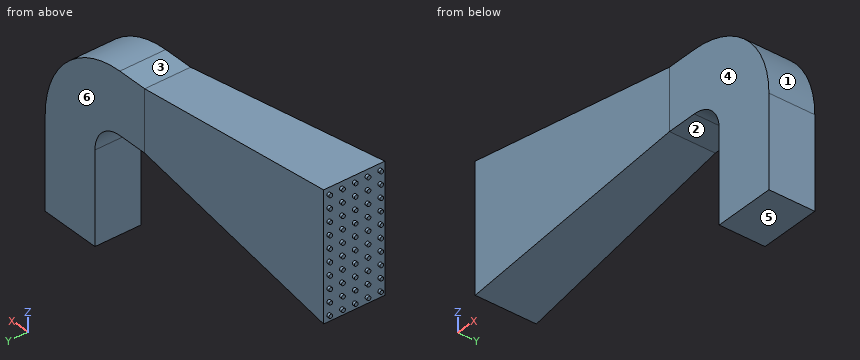
```python
from build123d import *

# Parameters (mm, degrees)
SKETCH_2_5_W    = 240
SKETCH_2_5_H    = 180
EXTRUDE_2_DEPTH = 120
SKETCH_10_W     = 240
SKETCH_10_H     = 180
REVOLVE_2_ANGLE = 90
SKETCH_11_W     = 240
SKETCH_11_H     = 180
EXTRUDE_3_DEPTH = 360
SKETCH_13_R     = 7.5
EXTRUDE_4_DEPTH = 10


with BuildPart() as part:
    # Sketch 2 → Loft 1 section 0
    with BuildSketch(Plane(origin=(900, 0, 0), x_dir=(0, 0, -1), z_dir=(1, 0, 0))):
        with BuildLine():
            Line((-120, 90), (120, 90))
            Line((120, 90), (120, -90))
            Line((120, -90), (-120, -90))
            Line((-120, -90), (-120, 90))
        make_face()
    # Sketch 1 → Loft 1 section 1
    with BuildSketch(Plane(origin=(0, 0, 0), x_dir=(0, 0, -1), z_dir=(1, 0, 0))):
        with BuildLine():
            Line((-250, 120), (250, 120))
            Line((250, 120), (250, -120))
            Line((250, -120), (-250, -120))
            Line((-250, -120), (-250, 120))
        make_face()
    loft()

    # Sketch 2_5 → Extrude 2 (add)
    with BuildSketch(Plane(origin=(900, 0, 0), x_dir=(0, 0, -1), z_dir=(1, 0, 0))):
        Rectangle(SKETCH_2_5_W, SKETCH_2_5_H)
    extrude(amount=EXTRUDE_2_DEPTH)

    # Sketch 10 → Revolve 2 (revolve)
    with BuildSketch(Plane(origin=(1020, 0, 0), x_dir=(0, 0, -1), z_dir=(1, 0, 0))):
        Rectangle(SKETCH_10_W, SKETCH_10_H)
    revolve(axis=Axis((1020, 90, -240), (0, 1, 0)), revolution_arc=REVOLVE_2_ANGLE)

    # Sketch 11 → Extrude 3 (add)
    with BuildSketch(Plane(origin=(0, 0, -240), x_dir=(-1, 0, 0), z_dir=(0, 0, -1))):
        with Locations((-1260, 0)):
            Rectangle(SKETCH_11_W, SKETCH_11_H)
    extrude(amount=EXTRUDE_3_DEPTH)

    # Sketch 13 → Extrude 4 (add)
    with BuildSketch(Plane.ZY):
        with Locations(Location((225, -100, 0), (0, 0, 180))):
            Circle(SKETCH_13_R)
        with Locations(Location((175, -100, 0), (0, 0, 180))):
            Circle(SKETCH_13_R)
        with Locations(Location((125, -100, 0), (0, 0, 180))):
            Circle(SKETCH_13_R)
        with Locations(Location((75, -100, 0), (0, 0, 180))):
            Circle(SKETCH_13_R)
        with Locations(Location((25, -100, 0), (0, 0, 180))):
            Circle(SKETCH_13_R)
        with Locations(Location((-25, -100, 0), (0, 0, 180))):
            Circle(SKETCH_13_R)
        with Locations(Location((-75, -100, 0), (0, 0, 180))):
            Circle(SKETCH_13_R)
        with Locations(Location((-125, -100, 0), (0, 0, 180))):
            Circle(SKETCH_13_R)
        with Locations(Location((-175, -100, 0), (0, 0, 180))):
            Circle(SKETCH_13_R)
        with Locations(Location((-225, -100, 0), (0, 0, 180))):
            Circle(SKETCH_13_R)
        with Locations(Location((175, -50, 0), (0, 0, 180))):
            Circle(SKETCH_13_R)
        with Locations(Location((125, -50, 0), (0, 0, 180))):
            Circle(SKETCH_13_R)
        with Locations(Location((75, -50, 0), (0, 0, 180))):
            Circle(SKETCH_13_R)
        with Locations(Location((25, -50, 0), (0, 0, 180))):
            Circle(SKETCH_13_R)
        with Locations(Location((-25, -50, 0), (0, 0, 180))):
            Circle(SKETCH_13_R)
        with Locations(Location((-75, -50, 0), (0, 0, 180))):
            Circle(SKETCH_13_R)
        with Locations(Location((-125, -50, 0), (0, 0, 180))):
            Circle(SKETCH_13_R)
        with Locations(Location((-175, -50, 0), (0, 0, 180))):
            Circle(SKETCH_13_R)
        with Locations(Location((-225, -50, 0), (0, 0, 180))):
            Circle(SKETCH_13_R)
        with Locations(Location((175, 0, 0), (0, 0, 180))):
            Circle(SKETCH_13_R)
        with Locations(Location((125, 0, 0), (0, 0, 180))):
            Circle(SKETCH_13_R)
        with Locations(Location((75, 0, 0), (0, 0, 180))):
            Circle(SKETCH_13_R)
        with Locations(Location((25, 0, 0), (0, 0, 180))):
            Circle(SKETCH_13_R)
        with Locations(Location((-25, 0, 0), (0, 0, 180))):
            Circle(SKETCH_13_R)
        with Locations(Location((-75, 0, 0), (0, 0, 180))):
            Circle(SKETCH_13_R)
        with Locations(Location((-125, 0, 0), (0, 0, 180))):
            Circle(SKETCH_13_R)
        with Locations(Location((-175, 0, 0), (0, 0, 180))):
            Circle(SKETCH_13_R)
        with Locations(Location((-225, 0, 0), (0, 0, 180))):
            Circle(SKETCH_13_R)
        with Locations(Location((175, 50, 0), (0, 0, 180))):
            Circle(SKETCH_13_R)
        with Locations(Location((125, 50, 0), (0, 0, 180))):
            Circle(SKETCH_13_R)
        with Locations(Location((75, 50, 0), (0, 0, 180))):
            Circle(SKETCH_13_R)
        with Locations(Location((25, 50, 0), (0, 0, 180))):
            Circle(SKETCH_13_R)
        with Locations(Location((-25, 50, 0), (0, 0, 180))):
            Circle(SKETCH_13_R)
        with Locations(Location((-75, 50, 0), (0, 0, 180))):
            Circle(SKETCH_13_R)
        with Locations(Location((-125, 50, 0), (0, 0, 180))):
            Circle(SKETCH_13_R)
        with Locations(Location((-175, 50, 0), (0, 0, 180))):
            Circle(SKETCH_13_R)
        with Locations(Location((-225, 50, 0), (0, 0, 180))):
            Circle(SKETCH_13_R)
        with Locations(Location((175, 100, 0), (0, 0, 180))):
            Circle(SKETCH_13_R)
        with Locations(Location((125, 100, 0), (0, 0, 180))):
            Circle(SKETCH_13_R)
        with Locations(Location((75, 100, 0), (0, 0, 180))):
            Circle(SKETCH_13_R)
        with Locations(Location((25, 100, 0), (0, 0, 180))):
            Circle(SKETCH_13_R)
        with Locations(Location((-25, 100, 0), (0, 0, 180))):
            Circle(SKETCH_13_R)
        with Locations(Location((-75, 100, 0), (0, 0, 180))):
            Circle(SKETCH_13_R)
        with Locations(Location((-125, 100, 0), (0, 0, 180))):
            Circle(SKETCH_13_R)
        with Locations(Location((-175, 100, 0), (0, 0, 180))):
            Circle(SKETCH_13_R)
        with Locations(Location((-225, 100, 0), (0, 0, 180))):
            Circle(SKETCH_13_R)
        with Locations(Location((225, -50, 0), (0, 0, 180))):
            Circle(SKETCH_13_R)
        with Locations(Location((225, 0, 0), (0, 0, 180))):
            Circle(SKETCH_13_R)
        with Locations(Location((225, 50, 0), (0, 0, 180))):
            Circle(SKETCH_13_R)
        with Locations(Location((225, 100, 0), (0, 0, 180))):
            Circle(SKETCH_13_R)
    extrude(amount=EXTRUDE_4_DEPTH)


solid = part.part
```
Geometry: final body of the model. Coordinates: model frame, mm. Face numbers are marked on the shaded views. A direction names the side the tool comes from. Give positions to 0.01 mm unless a question says otherwise; leave off trailing zeros. Loops run counter-clockwise (first coordinate to the right, second up) from the corner with the lowest first, then second, coordinate; pieces in that order, holes last. Notation, with made-up numbers: (87, -9.5) -> (114, -9.5) arc R13 cw to (114, 5.5) -> close; hole circle Ø3 at (2, 12.5). An arc over 180 degrees is marked (long way). Use one line per item in the form item = value.
Item 1: Access query for the marked faces 4, 5 and 6. Directions: +Z, -Z, +X, -X, +Y, -Y. A direction counts if a zero-diameter tool reaches every point of the face in a straight line with its end or side. Return the directions, or none.
A:
face_4 = +Z, -Z, +X, -Y
face_5 = -Z, +X, -X, +Y, -Y
face_6 = +Z, -Z, +X, +Y
Item 2: Section query B-B on x = 1170.5. Output: boundary loops of the cut face in (y, z).
A:
outline = (-90, -600) -> (90, -600) -> (90, 87.03) -> (-90, 87.03) -> close
Item 3: Pin query (flat end, axial travel): P1, Ø6, axis at y = -62, z = 57.5, coming from the +X side; P2, Ø8, axis at x = 544, y = 10.5, coming from the +Z side; P3, Ø4, axis at x = 1130.5, z = -131.5, coming from the +Y side. Return the tip coordinate at first contact, or that it passes through.
A:
P1 = 1227.05
P2 = 172
P3 = 90
Item 4: Line query: probe 1 along Y at (x, z) = (366, -155); probe 2 along Y at (x, z) = (1286.5, -177); probe 3 along X at (y, z) = (26.5, -399). Output: solid intervals per line, ascending.
A:
probe_1 = -107.8 to 107.8
probe_2 = -90 to 90
probe_3 = 1140 to 1380
Item 5: Section query A-A on z = -421. Output: boundary loops of the cut face in (x, y), and give its area (3 significant figures).
A:
outline = (1140, -90) -> (1380, -90) -> (1380, 90) -> (1140, 90) -> close
area = 43,200 mm^2
Item 6: Draft query along X for the marked faces 1, 2 and 3. Return one class per face: pulls with the +X half, pulls with the -X half, needs draft (parallel to the pull), parting line crosses it, or undercut.
A:
face_1 = pulls with the +X half
face_2 = undercut
face_3 = needs draft
